from build123d import *

# Parameters (mm, degrees)
SKETCH_1_W          = 70
SKETCH_1_H          = 100
SKETCH_1_R          = 1.6
EXTRUDE_1_DEPTH     = 4
SKETCH_2_W          = 15
SKETCH_2_H          = 3
SKETCH_2_W_2        = 25
EXTRUDE_2_DEPTH     = 82
SKETCH_3_R          = 1.5
SKETCH_3_R_2        = 1.539226355
CUT_EXTRUDE_1_DEPTH = 8
EXTRUDE_3_DEPTH     = 2
SKETCH_7_R          = 1.6
EXTRUDE_5_DEPTH     = 82
SKETCH_10_R         = 1.5
SKETCH_10_R_2       = 1.55
CUT_EXTRUDE_2_DEPTH = 118.749734607


with BuildPart() as part:
    # 草图1 → 凸台-拉伸1 (new body)
    with BuildSketch(Plane.XY):
        with Locations((3.334002404, 0)):
            Rectangle(SKETCH_1_W, SKETCH_1_H)
        with Locations((34.334002404, 26.5)):
            Circle(SKETCH_1_R, mode=Mode.SUBTRACT)
        with Locations((-16.665997596, -46)):
            Circle(SKETCH_1_R, mode=Mode.SUBTRACT)
        with Locations((3.334002404, 46)):
            Circle(SKETCH_1_R, mode=Mode.SUBTRACT)
        with Locations((10.834002404, 28.5)):
            Circle(SKETCH_1_R, mode=Mode.SUBTRACT)
        with Locations((10.834002404, -2.5)):
            Circle(SKETCH_1_R, mode=Mode.SUBTRACT)
        with Locations((34.334002404, -11.5)):
            Circle(SKETCH_1_R, mode=Mode.SUBTRACT)
        with Locations(Location((-27.665997596, 26.5, 0), (0, 0, 180))):
            Circle(SKETCH_1_R, mode=Mode.SUBTRACT)
        with Locations(Location((-4.165997596, 28.5, 0), (0, 0, 180))):
            Circle(SKETCH_1_R, mode=Mode.SUBTRACT)
        with Locations(Location((-4.165997596, -2.5, 0), (0, 0, 180))):
            Circle(SKETCH_1_R, mode=Mode.SUBTRACT)
        with Locations(Location((-27.665997596, -11.5, 0), (0, 0, 180))):
            Circle(SKETCH_1_R, mode=Mode.SUBTRACT)
        with Locations(Location((23.334002404, -46, 0), (0, 0, 180))):
            Circle(SKETCH_1_R, mode=Mode.SUBTRACT)
    extrude(amount=EXTRUDE_1_DEPTH)

    # 草图2 → 凸台-拉伸2 (add)
    with BuildSketch(Plane.XY.offset(4)):
        with Locations((-4.165997596, -19.5)):
            Rectangle(SKETCH_2_W, SKETCH_2_H)
        with Locations((15.834002404, -19.5)):
            Rectangle(SKETCH_2_W_2, SKETCH_2_H)
    extrude(amount=EXTRUDE_2_DEPTH)

    # 草图3 → 切除-拉伸1 (cut)
    with BuildSketch(Plane.XZ.offset(21)):
        with Locations(Location((-3.665997596, 83, 0), (0, 0, 270))):
            Circle(SKETCH_3_R)
        with Locations(Location((25.334002404, 83, 0), (0, 0, 90))):
            Circle(SKETCH_3_R)
        with Locations(Location((25.334002404, 29, 0), (0, 0, 270))):
            Circle(SKETCH_3_R)
        with Locations(Location((-3.665997596, 29, 0), (0, 0, 90))):
            Circle(SKETCH_3_R)
        with Locations(Location((8.334002404, 63, 0), (0, 0, 270))):
            Circle(SKETCH_3_R)
        with Locations(Location((8.334002404, 56, 0), (0, 0, 270))):
            Circle(SKETCH_3_R_2)
        with Locations(Location((15.334002404, 56, 0), (0, 0, 270))):
            Circle(SKETCH_3_R)
        with Locations(Location((8.334002404, 49, 0), (0, 0, 270))):
            Circle(SKETCH_3_R)
        with Locations(Location((1.334002404, 56, 0), (0, 0, 270))):
            Circle(SKETCH_3_R)
    extrude(amount=-CUT_EXTRUDE_1_DEPTH, mode=Mode.SUBTRACT)

    # 草图6 → 凸台-拉伸3 (add, symmetric)
    with BuildSketch(Plane.YZ.offset(8.334002404)):
        Polygon((-21, 44.617390455), (-36.570771874, 4), (-21, 4), align=None)
    extrude(amount=EXTRUDE_3_DEPTH, both=True)

    # 草图7 → 凸台-拉伸5 (add)
    with BuildSketch(Plane.XY.offset(4)):
        with Locations((34.334002404, -11.5)):
            Circle(SKETCH_7_R)
        Polygon((31.334002404, -21), (28.334002404, -21), (28.334002404, -18), (28.334002404, 9), (31.334002404, 9), align=None)
    extrude(amount=EXTRUDE_5_DEPTH)


with BuildPart() as extrude_5_kept_piece:
    # of the separate pieces the step leaves, the one the design keeps (extrude_5_pieces_kept)
    add(part.part.solids().sort_by_distance((-31.665997596, 50, 0))[0])

    # 草图10 → 切除-拉伸2 (cut, through all)
    with BuildSketch(Plane(origin=(31.334002404, 0, 0), x_dir=(0, 0, -1), z_dir=(1, 0, 0))):
        with Locations((-37, -12)):
            Circle(SKETCH_10_R)
        with Locations((-37, 6)):
            Circle(SKETCH_10_R)
        with Locations((-75, -12)):
            Circle(SKETCH_10_R)
        with Locations(Location((-75, 6, 0), (0, 0, 270))):
            Circle(SKETCH_10_R)
        with Locations((-56, -3)):
            Circle(SKETCH_10_R_2)
    extrude(amount=-CUT_EXTRUDE_2_DEPTH, mode=Mode.SUBTRACT)


solid = extrude_5_kept_piece.part
Work out the finished part from the listing and answer in its coordinate system (mm). A direction names the side the tool comes from. Round coordinates to 2 decimals unless told otherwise and drop trailing zeros. Write each loop counter-clockwise with the first axis right and the second up, starting at its lowest first coordinate (ties: lowest second). Pieces come first, ordered by that corner, then holes. Notation, with made-up numbers: (59.5, -17) - (75.5, -17) arc R26 ccw to (75.5, 15) - close; hole circle Ø4 at (-20, -12). An arc over 180 degrees is marked (long way). Answer in a Markdown table with one row per item. Add a question column.
1. The mould has two halves that part along Y. Classify faces 1 (the cylindrical face through (22.6, -44.58, 1.97)), 2 (the cylindrical face through (7.42, -19.52, 50.19)), 3 (the flat face through (3, -50, 2)): +Y half, -Y half, draft (parallel to the pull), parting line (faces both ways), or undercut.
2. A cutting plane is placed at A-A, the plane z = 83. Determine the outline of the cut face in (x, y).
3. A cutting plane is placed at D-D, the plane y = -29. Determine the outline of the cut face in (x, z), and give its area (3 significant figures).
4. A cutting plane is placed at C-C, the plane z = 29. Determine the outline of the cut face in (x, y).
5. Given pin 1 (3.5 mm diameter, centred on x = 10.83, y = -2.5, fed in from -Z); pin 2 (4 mm diameter, centred on y = 6, z = 37, fed in from -X); pin 3 (3.5 mm diameter, centred on x = -3.67, z = 83, fed in from -Y); pin 4 (10 mm diameter, centred on x = 20, y = 3.5, fed in from +Z), each flat-ended and moving along its own axis, determine where each tip first touches the part or whether it passes through.
6. For faces 4 (the flat face through (31.334, -6, 44)), 5 (the flat face through (14, -21, 44)), 6 (the flat face through (9, -18, 44)), 7 (the flat face through (-11.666, -20, 44)), 8 (the flat face through (3, 50, 2)), determine the directions among +Z, -Z, +X, -X, +Y, -Y from which every point of the face is accessible in a straight line to the end or side of a thin tool.
7. Find the intervals of material crossed by line 1 along X through (y, z) = (-19.35, 29); line 2 along Z through (x, y) = (-3.5, 0); line 3 along Y through (x, z) = (28, 22), in increasing order. Write a range as from..to.
8. A cutting plane is placed at B-B, the plane x = -19.5. Determine the outline of the cut face in (y, z), and give its area (3 significant figures).
Worked out:
| question | item | result |
|---|---|---|
| 1 | face 1 | undercut |
| 1 | face 2 | draft |
| 1 | face 3 | -Y half |
| 2 | outline | (-11.67, -21) - (-5.17, -21) - (-5.17, -18) - (-11.67, -18) - close; (-2.17, -21) - (23.83, -21) - (23.83, -18) - (-2.17, -18) - close; (26.83, -21) - (31.33, -21) - (31.33, 9) - (28.33, 9) - (28.33, -18) - (26.83, -18) - close |
| 3 | outline | (-31.67, 0) - (38.33, 0) - (38.33, 4) - (10.33, 4) - (10.33, 23.75) - (6.33, 23.75) - (6.33, 4) - (-31.67, 4) - close |
| 3 | area | 359 mm^2 |
| 4 | outline | (-11.67, -21) - (-5.17, -21) - (-5.17, -18) - (-11.67, -18) - close; (-2.17, -21) - (6.33, -21) - (6.33, -26.99) - (10.33, -26.99) - (10.33, -21) - (23.83, -21) - (23.83, -18) - (-2.17, -18) - close; (26.83, -21) - (31.33, -21) - (31.33, 9) - (28.33, 9) - (28.33, -18) - (26.83, -18) - close |
| 5 | pin 1 | z = 0 |
| 5 | pin 2 | x = 28.33 |
| 5 | pin 3 | y = -21 |
| 5 | pin 4 | z = 4 |
| 6 | face 4 | +Z, +X, +Y, -Y |
| 6 | face 5 | +Z, -Y |
| 6 | face 6 | +Z, -X, +Y |
| 6 | face 7 | +Z, -X, +Y, -Y |
| 6 | face 8 | +Z, -Z, +X, -X, +Y |
| 7 | line 1 | -11.67..-5.17, -2.17..23.83, 26.83..31.33 |
| 7 | line 2 | 0..4 |
| 7 | line 3 | -21..-18 |
| 8 | outline | (-50, 0) - (50, 0) - (50, 4) - (-50, 4) - close |
| 8 | area | 400 mm^2 |
